Design review of the part built by this model. Coordinates are the model's own, in mm. Face numbers are marked on the shaded views. Coordinates: 2 decimals unless noted, no trailing zeros. Write each loop counter-clockwise with the first axis right and the second up, starting at its lowest first coordinate (ties: lowest second). Pieces come first, ordered by that corner, then holes. Notation, with made-up numbers: (-27.75, 78) -> (-16.75, 78) arc R14 cw to (-16.75, 90) -> close; hole circle Ø2 at (89, -15). An arc over 180 degrees is marked (long way). Write item = value, one per line. Start each with the question number.
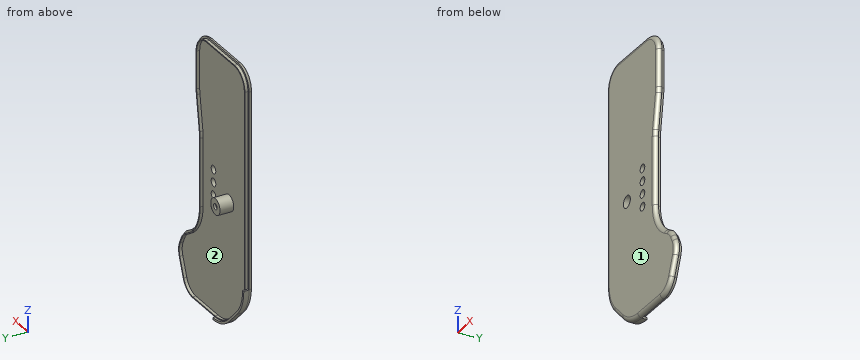
Autodesk Fusion 360 part; units mm, degrees
sketch "Sketch1" plane through (0, 0, 0) normal (0, 1, 0) x (1, 0, 0)
  line L0 (31.7101, -12.3063) -> (34.0314, -10.9136)
  arc A0 (39.2196, -4.033) -> (39.6234, 3.9906) centre (30.2753, 0.4391) ccw
  line L1 (37.8307, -6.8108) -> (39.2196, -4.033)
  arc A1 (15, -115) -> (25, -105) centre (15, -105) ccw
  arc A2 (31.7101, -12.3063) -> (22, -29.4562) centre (42, -29.4562) ccw
  arc A3 (34.0314, -10.9136) -> (37.8307, -6.8108) centre (28.8864, -2.3386) ccw
  arc A4 (36.181, 13.0515) -> (26.8329, 19.5) centre (26.8329, 9.5) ccw
  line L2 (39.6234, 3.9906) -> (36.181, 13.0515)
  arc A5 (-13.6421, 6.6863) -> (-19.5, -7.4558) centre (0.5, -7.4558) ccw
  line L3 (22, -63.3592) -> (22, -29.4562)
  arc A6 (7.4558, 19.5) -> (-6.6863, 13.6421) centre (7.4558, -0.5) ccw
  line L4 (24.7787, -83.3757) -> (22.2213, -66.326)
  arc A7 (25, -86.3425) -> (24.7787, -83.3757) centre (5, -86.3425) ccw
  line L5 (-6.6863, 13.6421) -> (-13.6421, 6.6863)
  line L6 (-9.5, -115) -> (15, -115)
  arc A8 (-19.5, -105) -> (-9.5, -115) centre (-9.5, -105) ccw
  line L7 (25, -105) -> (25, -86.3425)
  line L8 (26.8329, 19.5) -> (7.4558, 19.5)
  line L9 (-19.5, -7.4558) -> (-19.5, -105)
  arc A9 (22, -63.3592) -> (22.2213, -66.326) centre (42, -63.3592) ccw
extrude "Extrude1" add sketch "Sketch1" along normal blind 2
sketch "Sketch2" plane through (0, 2, 0) normal (0, 1, 0) x (-1, 0, 0)
  line L0 (-31.7101, 12.3063) -> (-34.0314, 10.9136)
  arc A0 (-34.0314, 10.9136) -> (-37.8307, 6.8108) centre (-28.8864, 2.3386) ccw
  line L1 (-37.8307, 6.8108) -> (-39.2196, 4.033)
  arc A1 (-39.2196, 4.033) -> (-39.6234, -3.9906) centre (-30.2753, -0.4391) ccw
  line L2 (-39.6234, -3.9906) -> (-36.181, -13.0515)
  arc A2 (-36.181, -13.0515) -> (-26.8329, -19.5) centre (-26.8329, -9.5) ccw
  line L3 (-26.8329, -19.5) -> (-7.4558, -19.5)
  arc A3 (-7.4558, -19.5) -> (6.6863, -13.6421) centre (-7.4558, 0.5) ccw
  line L4 (6.6863, -13.6421) -> (13.6421, -6.6863)
  arc A4 (13.6421, -6.6863) -> (19.5, 7.4558) centre (-0.5, 7.4558) ccw
  line L5 (19.5, 7.4558) -> (19.5, 105)
  arc A5 (19.5, 105) -> (9.5, 115) centre (9.5, 105) ccw
  line L6 (9.5, 115) -> (-15, 115)
  arc A6 (-15, 115) -> (-25, 105) centre (-15, 105) ccw
  line L7 (-25, 105) -> (-25, 86.3425)
  arc A7 (-25, 86.3425) -> (-24.7787, 83.3757) centre (-5, 86.3425) ccw
  line L8 (-24.7787, 83.3757) -> (-22.2213, 66.326)
  arc A8 (-22, 63.3592) -> (-22.2213, 66.326) centre (-42, 63.3592) ccw
  line L9 (-22, 63.3592) -> (-22, 29.4562)
  arc A9 (-31.7101, 12.3063) -> (-22, 29.4562) centre (-42, 29.4562) ccw
  line L10 (18.5, 7.4558) -> (18.5, 105)
  arc A10 (18.5, 105) -> (9.5, 114) centre (9.5, 105) ccw
  line L11 (9.5, 114) -> (-15, 114)
  arc A11 (-15, 114) -> (-24, 105) centre (-15, 105) ccw
  line L12 (-24, 105) -> (-24, 86.3425)
  arc A12 (-24, 86.3425) -> (-23.7898, 83.524) centre (-5, 86.3425) ccw
  line L13 (-23.7898, 83.524) -> (-21.2323, 66.4743)
  arc A13 (-21, 63.3592) -> (-21.2323, 66.4743) centre (-42, 63.3592) ccw
  line L14 (-21, 63.3592) -> (-21, 29.4562)
  arc A14 (-31.1956, 11.4488) -> (-21, 29.4562) centre (-42, 29.4562) ccw
  line L15 (-31.1956, 11.4488) -> (-33.5169, 10.0561)
  arc A15 (-33.5169, 10.0561) -> (-36.9363, 6.3636) centre (-28.8864, 2.3386) ccw
  line L16 (-36.9363, 6.3636) -> (-38.3251, 3.5858)
  arc A16 (-38.3251, 3.5858) -> (-38.6886, -3.6354) centre (-30.2753, -0.4391) ccw
  line L17 (-38.6886, -3.6354) -> (-35.2462, -12.6963)
  arc A17 (-35.2462, -12.6963) -> (-26.8329, -18.5) centre (-26.8329, -9.5) ccw
  line L18 (-26.8329, -18.5) -> (-7.4558, -18.5)
  arc A18 (-7.4558, -18.5) -> (5.9792, -12.935) centre (-7.4558, 0.5) ccw
  line L19 (5.9792, -12.935) -> (12.935, -5.9792)
  arc A19 (12.935, -5.9792) -> (18.5, 7.4558) centre (-0.5, 7.4558) ccw
  line L20 (9.5, 113.5) -> (-15, 113.5)
  arc A20 (-15, 113.5) -> (-23.5, 105) centre (-15, 105) ccw
  line L21 (-23.5, 105) -> (-23.5, 86.3425)
  arc A21 (-23.5, 86.3425) -> (-23.2953, 83.5982) centre (-5, 86.3425) ccw
  line L22 (-23.2953, 83.5982) -> (-20.7379, 66.5485)
  arc A22 (-20.5, 63.3592) -> (-20.7379, 66.5485) centre (-42, 63.3592) ccw
  line L23 (-20.5, 63.3592) -> (-20.5, 29.4562)
  arc A23 (-30.9383, 11.0201) -> (-20.5, 29.4562) centre (-42, 29.4562) ccw
  line L24 (-30.9383, 11.0201) -> (-33.2596, 9.6273)
  arc A24 (-33.2596, 9.6273) -> (-36.489, 6.1399) centre (-28.8864, 2.3386) ccw
  line L25 (-36.489, 6.1399) -> (-37.8779, 3.3622)
  arc A25 (-37.8779, 3.3622) -> (-38.2212, -3.4579) centre (-30.2753, -0.4391) ccw
  line L26 (-38.2212, -3.4579) -> (-34.7788, -12.5188)
  arc A26 (-34.7788, -12.5188) -> (-26.8329, -18) centre (-26.8329, -9.5) ccw
  line L27 (-26.8329, -18) -> (-7.4558, -18)
  arc A27 (-7.4558, -18) -> (5.6256, -12.5815) centre (-7.4558, 0.5) ccw
  line L28 (5.6256, -12.5815) -> (12.5815, -5.6256)
  arc A28 (12.5815, -5.6256) -> (18, 7.4558) centre (-0.5, 7.4558) ccw
  line L29 (18, 7.4558) -> (18, 105)
  arc A29 (18, 105) -> (9.5, 113.5) centre (9.5, 105) ccw
  dimension "d40" = -1
  dimension "d41" = -1.5
extrude "Extrude2" add sketch "Sketch2" along normal blind 1.5 contours L10 A10 L11 A11 L12 A12 L13 A13 L14 A14 L15 A15 L16 A16 L17 A17 L18 A18 L19 A19
sketch "Sketch3" plane through (0, 2, 0) normal (0, 1, 0) x (-1, 0, 0)
  line L0 (19.5, 7.4558) -> (18.5, 7.4558)
  arc A0 (-31.7101, 12.3063) -> (-22, 29.4562) centre (-42, 29.4562) ccw
  line L1 (-31.7101, 12.3063) -> (-34.0314, 10.9136)
  arc A1 (-34.0314, 10.9136) -> (-37.8307, 6.8108) centre (-28.8864, 2.3386) ccw
  line L2 (-37.8307, 6.8108) -> (-39.2196, 4.033)
  line L3 (-25, 105) -> (-25, 86.3425)
  arc A2 (-25, 86.3425) -> (-24.7787, 83.3757) centre (-5, 86.3425) ccw
  line L4 (-24.7787, 83.3757) -> (-22.2213, 66.326)
  arc A3 (-22, 63.3592) -> (-22.2213, 66.326) centre (-42, 63.3592) ccw
  line L5 (-22, 63.3592) -> (-22, 29.4562)
  line L6 (-39.6234, -3.9906) -> (-36.181, -13.0515)
  arc A4 (-36.181, -13.0515) -> (-26.8329, -19.5) centre (-26.8329, -9.5) ccw
  line L7 (-26.8329, -19.5) -> (-7.4558, -19.5)
  arc A5 (-7.4558, -19.5) -> (6.6863, -13.6421) centre (-7.4558, 0.5) ccw
  line L8 (6.6863, -13.6421) -> (13.6421, -6.6863)
  arc A6 (13.6421, -6.6863) -> (19.5, 7.4558) centre (-0.5, 7.4558) ccw
  line L9 (19.5, 7.4558) -> (19.5, 105)
  arc A7 (19.5, 105) -> (9.5, 115) centre (9.5, 105) ccw
  line L10 (9.5, 115) -> (-15, 115)
  arc A8 (-15, 115) -> (-25, 105) centre (-15, 105) ccw
  arc A9 (-33.2596, 9.6273) -> (-36.489, 6.1399) centre (-28.8864, 2.3386) ccw
  line L11 (-36.489, 6.1399) -> (-37.8779, 3.3622)
  arc A10 (-37.8779, 3.3622) -> (-38.2212, -3.4579) centre (-30.2753, -0.4391) ccw
  line L12 (-38.2212, -3.4579) -> (-34.7788, -12.5188)
  arc A11 (-34.7788, -12.5188) -> (-26.8329, -18) centre (-26.8329, -9.5) ccw
  line L13 (-26.8329, -18) -> (-7.4558, -18)
  arc A12 (-7.4558, -18) -> (5.6256, -12.5815) centre (-7.4558, 0.5) ccw
  line L14 (5.6256, -12.5815) -> (12.5815, -5.6256)
  arc A13 (12.5815, -5.6256) -> (18, 7.4558) centre (-0.5, 7.4558) ccw
  line L15 (18, 7.4558) -> (18, 105)
  arc A14 (18, 105) -> (9.5, 113.5) centre (9.5, 105) ccw
  line L16 (9.5, 113.5) -> (-15, 113.5)
  arc A15 (-15, 113.5) -> (-23.5, 105) centre (-15, 105) ccw
  line L17 (-23.5, 105) -> (-23.5, 86.3425)
  arc A16 (-23.5, 86.3425) -> (-23.2953, 83.5982) centre (-5, 86.3425) ccw
  line L18 (-23.2953, 83.5982) -> (-20.7379, 66.5485)
  arc A17 (-20.5, 63.3592) -> (-20.7379, 66.5485) centre (-42, 63.3592) ccw
  line L19 (-20.5, 63.3592) -> (-20.5, 29.4562)
  arc A18 (-30.9383, 11.0201) -> (-20.5, 29.4562) centre (-42, 29.4562) ccw
  line L20 (-30.9383, 11.0201) -> (-33.2596, 9.6273)
  arc A19 (-39.2196, 4.033) -> (-39.6234, -3.9906) centre (-30.2753, -0.4391) ccw
  arc A20 (-31.1956, 11.4488) -> (-21, 29.4562) centre (-42, 29.4562) ccw
  line L21 (-21, 29.4562) -> (-21, 63.3592)
  arc A21 (-21, 63.3592) -> (-21.2323, 66.4743) centre (-42, 63.3592) ccw
  line L22 (-21.2323, 66.4743) -> (-23.7898, 83.524)
  arc A22 (-24, 86.3425) -> (-23.7898, 83.524) centre (-5, 86.3425) ccw
  line L23 (-24, 86.3425) -> (-24, 105)
  arc A23 (-15, 114) -> (-24, 105) centre (-15, 105) ccw
  line L24 (-15, 114) -> (9.5, 114)
  arc A24 (18.5, 105) -> (9.5, 114) centre (9.5, 105) ccw
  line L25 (18.5, 105) -> (18.5, 7.4558)
  arc A25 (12.935, -5.9792) -> (18.5, 7.4558) centre (-0.5, 7.4558) ccw
  line L26 (12.935, -5.9792) -> (5.9792, -12.935)
  arc A26 (-7.4558, -18.5) -> (5.9792, -12.935) centre (-7.4558, 0.5) ccw
  line L27 (-7.4558, -18.5) -> (-26.8329, -18.5)
  arc A27 (-35.2462, -12.6963) -> (-26.8329, -18.5) centre (-26.8329, -9.5) ccw
  line L28 (-35.2462, -12.6963) -> (-38.6886, -3.6354)
  arc A28 (-38.3251, 3.5858) -> (-38.6886, -3.6354) centre (-30.2753, -0.4391) ccw
  line L29 (-38.3251, 3.5858) -> (-36.9363, 6.3636)
  arc A29 (-33.5169, 10.0561) -> (-36.9363, 6.3636) centre (-28.8864, 2.3386) ccw
  line L30 (-33.5169, 10.0561) -> (-31.1956, 11.4488)
  line L31 (-7.4558, -18.5) -> (-7.4558, -19.5)
extrude "Extrude3" add sketch "Sketch3" along normal blind 2.6 contours L0 A5 L8 A6 A25 L26 A26 L31
sketch "Sketch4" plane through (0, 0, 0) normal (0, -1, 0) x (1, 0, 0)
  circle A0 centre (11.5, 33) radius 2
  circle A1 centre (11.5, 39.3) radius 2
  circle A2 centre (11.5, 45.6) radius 2
  circle A3 centre (11.5, 51.9) radius 2
  line L0 (34.0314, 10.9136) -> (31.7101, 12.3063)
  arc A4 (22, 29.4562) -> (31.7101, 12.3063) centre (42, 29.4562) ccw
  line L1 (22, 29.4562) -> (22, 63.3592)
  arc A5 (22.2213, 66.326) -> (22, 63.3592) centre (42, 63.3592) ccw
  line L2 (22.2213, 66.326) -> (24.7787, 83.3757)
  arc A6 (24.7787, 83.3757) -> (25, 86.3425) centre (5, 86.3425) ccw
  line L3 (25, 86.3425) -> (25, 105)
  arc A7 (25, 105) -> (15, 115) centre (15, 105) ccw
  line L4 (15, 115) -> (-9.5, 115)
  arc A8 (-9.5, 115) -> (-19.5, 105) centre (-9.5, 105) ccw
  line L5 (-19.5, 105) -> (-19.5, 7.4558)
  arc A9 (-19.5, 7.4558) -> (-13.6421, -6.6863) centre (0.5, 7.4558) ccw
  line L6 (-13.6421, -6.6863) -> (-6.6863, -13.6421)
  arc A10 (-6.6863, -13.6421) -> (7.4558, -19.5) centre (7.4558, 0.5) ccw
  line L7 (7.4558, -19.5) -> (26.8329, -19.5)
  arc A11 (26.8329, -19.5) -> (36.181, -13.0515) centre (26.8329, -9.5) ccw
  line L8 (36.181, -13.0515) -> (39.6234, -3.9906)
  arc A12 (39.6234, -3.9906) -> (39.2196, 4.033) centre (30.2753, -0.4391) ccw
  line L9 (39.2196, 4.033) -> (37.8307, 6.8108)
  arc A13 (37.8307, 6.8108) -> (34.0314, 10.9136) centre (28.8864, 2.3386) ccw
  dimension "d14" = 4
  dimension "d18" = 0
  dimension "d19" = 6.3
  dimension "d44" = 10.5
extrude "Extrude4" cut sketch "Sketch4" against normal blind 5 contours A0 | A1 | A2 | A3
sketch "Sketch5" plane through (0, 2, 0) normal (0, 1, 0) x (-1, 0, 0)
  circle A0 centre (-11.5, 39.3) radius 2
  circle A1 centre (-11.5, 45.6) radius 2
  circle A2 centre (-11.5, 33) radius 2
  circle A3 centre (-11.5, 51.9) radius 2
  circle A4 centre (2.08, 42.036) radius 3
  circle A5 centre (2.08, 42.036) radius 4
  arc A6 (-33.2596, 9.6273) -> (-36.489, 6.1399) centre (-28.8864, 2.3386) ccw
  line L0 (-36.489, 6.1399) -> (-37.8779, 3.3622)
  arc A7 (-37.8779, 3.3622) -> (-38.2212, -3.4579) centre (-30.2753, -0.4391) ccw
  line L1 (-38.2212, -3.4579) -> (-34.7788, -12.5188)
  arc A8 (-34.7788, -12.5188) -> (-26.8329, -18) centre (-26.8329, -9.5) ccw
  line L2 (-26.8329, -18) -> (-7.4558, -18)
  arc A9 (-7.4558, -18) -> (5.6256, -12.5815) centre (-7.4558, 0.5) ccw
  line L3 (5.6256, -12.5815) -> (12.5815, -5.6256)
  arc A10 (12.5815, -5.6256) -> (18, 7.4558) centre (-0.5, 7.4558) ccw
  line L4 (18, 7.4558) -> (18, 105)
  arc A11 (18, 105) -> (9.5, 113.5) centre (9.5, 105) ccw
  arc A12 (-15, 113.5) -> (-23.5, 105) centre (-15, 105) ccw
  line L5 (-23.5, 105) -> (-23.5, 86.3425)
  arc A13 (-23.5, 86.3425) -> (-23.2953, 83.5982) centre (-5, 86.3425) ccw
  line L6 (-23.2953, 83.5982) -> (-20.7379, 66.5485)
  arc A14 (-20.5, 63.3592) -> (-20.7379, 66.5485) centre (-42, 63.3592) ccw
  line L7 (-20.5, 63.3592) -> (-20.5, 29.4562)
  arc A15 (-30.9383, 11.0201) -> (-20.5, 29.4562) centre (-42, 29.4562) ccw
  line L8 (-30.9383, 11.0201) -> (-33.2596, 9.6273)
  line L9 (19.5, 7.4558) -> (19.5, 105)
  line L10 (9.5, 115) -> (-15, 115)
  dimension "d22" = 6
  dimension "d23" = 8
  dimension "d42" = 17.42
  dimension "d43" = 72.964
extrude "Extrude5" add sketch "Sketch5" along normal blind 6.8 contours A5
extrude "Extrude6" cut 1 faces at (-1.2923, 2, 40.6272) along direction (0, -1, 0) blind 5
sketch "Sketch6" plane through (0, 8.8, 0) normal (0, 1, 0) x (-1, 0, 0)
  circle A0 centre (2.08, 42.036) radius 3
  circle A1 centre (2.08, 42.036) radius 4
  circle A2 centre (2.08, 42.036) radius 4
extrude "Extrude7" add sketch "Sketch6" against normal blind 1 contours A0 | A1 A2
sketch "Sketch7" plane through (0, 8.8, 0) normal (0, 1, 0) x (-1, 0, 0)
  circle A0 centre (2.08, 42.036) radius 4
  circle A1 centre (2.08, 42.036) radius 1.5
  dimension "d31" = 3
extrude "Extrude8" cut sketch "Sketch7" against normal blind 5 contours A1
fillet "Fillet1" radius 2 20 edges at (23.5, 0, 74.8508) (22.0554, 0, 64.8467) (22, 0, 46.4077) (24.596, 0, 19.6022) (32.8707, 0, 11.6099) (36.2236, 0, 9.1331) (38.5251, 0, 5.4219) (40.2626, 0, 0.0635) (37.9022, 0, -8.521) (32.5112, 0, -17.7315) (17.1444, 0, -19.5) (-0.1978, 0, -17.9776) (-10.1642, 0, -10.1642) (-17.9776, 0, -0.1978) (-19.5, 0, 56.2279) (-16.5711, 0, 112.0711) (2.75, 0, 115) (22.0711, 0, 112.0711) (25, 0, 95.6712) (24.9446, 0, 84.855)
(1) For line 1 (Z direction, x = -2.08, y = 8.1); line 2 (Z direction, x = 11.5, y = 1.6); line 3 (Z direction, x = 11.5, y = 0.5), list the stretches that pass through material, from the lowest coordinate up.
(2) For pin 1 Ø5 at (x, z) = (-2.08, 42.036) entering from +Y; pin 2 Ø5 at (x, z) = (-2.08, 42.036) entering from -Y; pin 3 Ø1.2 at (y, z) = (3, 50) entering from +X; pin 4 Ø0.8 at (x, y) = (-2, 2.5) entering from -Z, all flat-tipped, find the tip position at first contact; note any pin that passes through.
(3) Take a section at A-A, the plane x = 11.5. Count the separate pieces of the cut face and the enclosed holes in it, then the cut area to 3 significant figures.
(4) Mouldability with a two-part tool opening along Z and no side actions: class the marked faces 1 and 2 as pulls with the +Z half, pulls with the -Z half, needs draft (parallel to the pull), parting line crosses it, or undercut.
(5) Take a section at D-D, the plane y = 6.25. State the section outline as (x, z) points.
Report:
q1.line_1 = 38.04 to 40.54, 43.54 to 46.04
q1.line_2 = -19.46 to 31, 35 to 37.3, 41.3 to 43.6, 47.6 to 49.9, 53.9 to 114.96
q1.line_3 = -18.82 to 31, 35 to 37.3, 41.3 to 43.6, 47.6 to 49.9, 53.9 to 114.32
q2.pin_1 = 8.8
q2.pin_2 = 7.8
q2.pin_3 = 21
q2.pin_4 = -17.33
q3.separate_pieces = 5
q3.enclosed_holes = 0
q3.area = 237 mm2
q4.face_1 = needs draft
q4.face_2 = undercut
q5.outline = circle Ø8 at (-2.08, 42.04); hole circle Ø6 at (-2.08, 42.04)
